```python
from build123d import *

# Parameters (mm, degrees)
SKETCH1_W                = 28.8
SKETCH1_H                = 15.9
BOSS_EXTRUDE2_DEPTH      = 10.2
SKETCH3_R                = 1.45
CUT_EXTRUDE1_DEPTH       = 17.45
SKETCH7_R                = 1.5
BOSS_EXTRUDE6_DEPTH      = 3.2
BOSS_EXTRUDE6_DEPTH_BACK = 3.2
BOSS_EXTRUDE7_DEPTH      = 3.4
BOSS_EXTRUDE7_DEPTH_BACK = 3.4
SKETCH9_W                = 14.4
SKETCH9_H                = 0.8
BOSS_EXTRUDE8_DEPTH      = 3
BOSS_EXTRUDE8_DEPTH_BACK = 3


with BuildPart() as part:
    # Sketch1 → Boss-Extrude2 (new body)
    with BuildSketch(Plane(origin=(0, 0, 0), x_dir=(1, 0, 0), z_dir=(0, 1, 0))):
        Rectangle(SKETCH1_W, SKETCH1_H)
    extrude(amount=BOSS_EXTRUDE2_DEPTH)

    # Sketch3 → Cut-Extrude1 (cut)
    with BuildSketch(Plane(origin=(0, 10.2, 0), x_dir=(1, 0, 0), z_dir=(0, 1, 0))):
        with Locations((11.95, 5.15)):
            Circle(SKETCH3_R)
        with Locations((-10.25, -5.15)):
            Circle(SKETCH3_R)
    extrude(amount=-CUT_EXTRUDE1_DEPTH, mode=Mode.SUBTRACT)



with BuildPart() as body_2:
    # Sketch7 → Boss-Extrude6 (new body, two sides)
    with BuildSketch(Plane(origin=(0, 5.1, 0), x_dir=(1, 0, 0), z_dir=(0, 1, 0))) as boss_extrude6_sk:
        with Locations((-8.65, 13.95)):
            Circle(SKETCH7_R)
    extrude(amount=BOSS_EXTRUDE6_DEPTH)
    extrude(boss_extrude6_sk.sketch, amount=-BOSS_EXTRUDE6_DEPTH_BACK)


with BuildPart() as part_1:
    add(part.part)

    add(body_2.part)  # Boss-Extrude7 merges body 2
    # Sketch8 → Boss-Extrude7 (add, two sides)
    with BuildSketch(Plane(origin=(0, 5.1, 0), x_dir=(1, 0, 0), z_dir=(0, 1, 0))) as boss_extrude7_sk:
        with BuildLine():
            ThreePointArc((-7.45, 13.95), (-8.65, 15.15), (-9.85, 13.95))
            Line((-9.85, 13.95), (-9.85, 10.05))
            Line((-9.85, 10.05), (-9.85, 9.648933868))
            Line((-9.85, 9.648933868), (-8.65, 9.648933868))
            Line((-8.65, 9.648933868), (-7.45, 9.648933868))
            Line((-7.45, 9.648933868), (3.238900305, 9.648933868))
            Line((3.238900305, 9.648933868), (3.238900305, 7.95))
            Line((3.238900305, 7.95), (3.75, 7.95))
            Line((3.75, 7.95), (3.75, 9.648933868))
            Line((3.75, 9.648933868), (3.75, 10.05))
            Line((3.75, 10.05), (3.238900305, 10.05))
            Line((3.238900305, 10.05), (-7.45, 10.05))
            Line((-7.45, 10.05), (-7.45, 13.95))
        make_face()
    extrude(amount=BOSS_EXTRUDE7_DEPTH)
    extrude(boss_extrude7_sk.sketch, amount=-BOSS_EXTRUDE7_DEPTH_BACK)

    # Sketch9 → Boss-Extrude8 (add, two sides)
    with BuildSketch(Plane(origin=(0, 5.1, 0), x_dir=(1, 0, 0), z_dir=(0, 1, 0))) as boss_extrude8_sk:
        with Locations((21.6, 3.25)):
            Rectangle(SKETCH9_W, SKETCH9_H)
        with Locations((21.6, -4.85)):
            Rectangle(SKETCH9_W, SKETCH9_H)
        Polygon((0, -7.95), (0, -13.05), (11.95, -13.05), (11.95, -12.093699041), (0.986707236, -12.093699041), (0.986707236, -7.95), align=None)
    extrude(amount=BOSS_EXTRUDE8_DEPTH)
    extrude(boss_extrude8_sk.sketch, amount=-BOSS_EXTRUDE8_DEPTH_BACK)


solid = part_1.part
```
The model under review builds one solid part; all positions refer to its coordinate system, in mm. A direction names the side the tool comes from. Coordinates: 2 decimals unless noted, no trailing zeros. Write each loop counter-clockwise with the first axis right and the second up, starting at its lowest first coordinate (ties: lowest second). Pieces come first, ordered by that corner, then holes. Notation, with made-up numbers: (-36.5, 10.5) - (-9.5, 10.5) arc R16 ccw to (-9.5, 21.5) - close; hole circle Ø10 at (-38.5, 57). An arc over 180 degrees is marked (long way). Write item = value, one per line.
(1) Consider section A-A, the plane x = -1. Give the boundary of the cut face in (y, z), then the cut area to 3 significant figures.
Result sheet:
outline = (0, -7.95) - (10.2, -7.95) - (10.2, 7.95) - (0, 7.95) - close; (1.7, -10.05) - (8.5, -10.05) - (8.5, -9.65) - (1.7, -9.65) - close
area = 165 mm^2
(2) For P1, Ø4, axis at y = 7.5, z = -5.5, coming from the +X side; P2, Ø5, axis at x = -6, y = 3.5, coming from the +Z side; P3, Ø2.5, axis at y = 5, z = 9.5, coming from the -X side; P4, Ø1, axis at x = 5.5, y = 8.5, coming from the -Z side, all flat-tipped, find the tip position at first contact; note any pin that passes through.
Result sheet:
P1 = 28.8
P2 = 7.95
P3 = 0
P4 = -7.95
(3) For line 1 (X direction, y = 7.75, z = -5.15); line 2 (X direction, y = 6, z = 5.15); line 3 (Z direction, x = -10.25, y = 4.25), list the stretches that pass through material, from the lowest coordinate up. Write a range as [from, to].
Result sheet:
line_1 = [-14.4, 10.5], [13.4, 14.4]
line_2 = [-14.4, -11.7], [-8.8, 28.8]
line_3 = [-7.95, 3.7], [6.6, 7.95]
(4) Consider section D-D, the plane x = -8. Give the boundary of the cut face in (y, z), then the cut area to 3 significant figures.
Result sheet:
outline = (0, -7.95) - (10.2, -7.95) - (10.2, 7.95) - (0, 7.95) - close; (1.7, -14.96) - (1.9, -14.96) - (1.9, -15.3) - (8.3, -15.3) - (8.3, -14.96) - (8.5, -14.96) - (8.5, -9.65) - (1.7, -9.65) - close
area = 200 mm^2
(5) Consider section C-C, the plane z = -6. Give the boundary of the cut face in (x, y).
Result sheet:
outline = (-14.4, 0) - (10.78, 0) - (10.78, 10.2) - (-14.4, 10.2) - close; (13.12, 0) - (14.4, 0) - (14.4, 10.2) - (13.12, 10.2) - close
(6) Machinability: for faces 3 (the face through (-8, 1.7, -11)), 4 (the face through (4.2, 8.1, 12.4)), 5 (the face through (21, 5, -2.85)), 6 (the face through (11.95, 5.1, 12.6)), 7 (the face through (21, 8.1, 5)), which of the approach directions +Z, -Z, +X, -X, +Y, -Y give a long, thin tool a straight path to every point of the face, cutting with its end or side? Answer none if there is none.
Result sheet:
face_3 = -Z, +X, -X, -Y
face_4 = +Z, +X, -X, +Y
face_5 = +X, +Y, -Y
face_6 = +Z, +X, +Y, -Y
face_7 = +Z, -Z, +X, +Y
(7) Mouldability with a two-part tool opening along Z and no side actions: class faces 1 (the face through (28.8, 5, 5)), 2 (the face through (-0.2, 5, 7.95)) as pulls with the +Z half, pulls with the -Z half, needs draft (parallel to the pull), parting line crosses it, or undercut.
Result sheet:
face_1 = needs draft
face_2 = undercut
(8) Consider section B-B, the plane y = 3. Give the boundary of the cut face in (x, z), then the cut area to 3 significant figures.
Result sheet:
outline = (-14.4, -7.95) - (3.24, -7.95) - (3.24, -9.65) - (-9.85, -9.65) - (-9.85, -13.05) arc R1.5 ccw (long way) to (-7.45, -13.05) - (-7.45, -10.05) - (3.75, -10.05) - (3.75, -7.95) - (14.4, -7.95) - (14.4, -3.65) - (28.8, -3.65) - (28.8, -2.85) - (14.4, -2.85) - (14.4, 4.45) - (28.8, 4.45) - (28.8, 5.25) - (14.4, 5.25) - (14.4, 7.95) - (0.99, 7.95) - (0.99, 12.09) - (11.95, 12.09) - (11.95, 13.05) - (0, 13.05) - (0, 7.95) - (-14.4, 7.95) - close; hole circle Ø2.9 at (-10.25, 5.15); hole circle Ø2.9 at (11.95, -5.15)
area = 503 mm^2
